Here's how the part is built. I have some questions about the finished solid (model axes, mm). Round coordinates to 2 decimals unless told otherwise and drop trailing zeros. Order: outer loops, then holes, each group sorted by start corner. A loop starts at its lowest first (then second) coordinate and runs counter-clockwise, first axis right, second up. Notation, with made-up numbers: (55.5, 85.25) -> (67.5, 85.25) arc R26 ccw to (67.5, 114.25) -> close; hole circle Ø3 at (14.5, -13). An arc over 180 degrees is marked (long way). Answer in a Markdown table with one row per item.
```python
from build123d import *

# Parameters (mm, degrees)
SKETCH1_W           = 16
SKETCH1_H           = 20
BOSS_EXTRUDE1_DEPTH = 4.2
SKETCH2_R           = 2.25
CUT_EXTRUDE1_DEPTH  = 26.954575704
FILLET1_R           = 8


with BuildPart() as part:
    # Sketch1 → Boss-Extrude1 (new body)
    with BuildSketch(Plane.XY):
        with Locations((8, 10)):
            Rectangle(SKETCH1_W, SKETCH1_H)
    extrude(amount=BOSS_EXTRUDE1_DEPTH)

    # Sketch2 → Cut-Extrude1 (cut, through all)
    with BuildSketch(Plane.XY.offset(4.2)):
        with Locations((8, 10.8)):
            Circle(SKETCH2_R)
    extrude(amount=-CUT_EXTRUDE1_DEPTH, mode=Mode.SUBTRACT)

    # Fillet1
    fillet1_edges = [part.edges().sort_by_distance(p)[0] for p in [
        (16, 20, 2.1),
        (0, 20, 2.1),
    ]]
    fillet(fillet1_edges, radius=FILLET1_R - 0.0001)  # a hair under: the kernel refuses the full size


solid = part.part
```
1. Suppose I cut it at C-C on x = 6.5. Write out the boundary of the cut face in (y, z).
Numbers:
| item | result |
|---|---|
| outline | (0, 0) -> (9.12, 0) -> (9.12, 4.2) -> (0, 4.2) -> close; (12.48, 0) -> (19.86, 0) -> (19.86, 4.2) -> (12.48, 4.2) -> close |
2. We'd pull the mould along X, two halves only. Please class faces 1 (the face through (8, 8, 4.2)), 2 (the face through (6.34, 12.32, 2.13)), 3 (the face through (2.281, 17.594, 2.129)): released by +X, released by -X, zero draft, split by the parting line, or undercut.
Numbers:
| item | result |
|---|---|
| face 1 | zero draft |
| face 2 | undercut |
| face 3 | released by -X |
3. Suppose I cut it at A-A on y = 10.8. Write out the boundary of the cut face in (x, z).
Numbers:
| item | result |
|---|---|
| outline | (0, 0) -> (5.75, 0) -> (5.75, 4.2) -> (0, 4.2) -> close; (10.25, 0) -> (16, 0) -> (16, 4.2) -> (10.25, 4.2) -> close |
4. Suppose I cut it at D-D on y = 17.5. Write out the boundary of the cut face in (x, z).
Numbers:
| item | result |
|---|---|
| outline | (2.19, 0) -> (13.81, 0) -> (13.81, 4.2) -> (2.19, 4.2) -> close |
5. Please list where these lines run through material, in increasing order: line 1 along Y through (x, z) = (8, 3.1); line 2 along Y through (x, z) = (10, 0.3); line 3 along Y through (x, z) = (12.25, 1.75).
Numbers:
| item | result |
|---|---|
| line 1 | y = 0 to 8.55, 13.05 to 20 |
| line 2 | y = 0 to 9.77, 11.83 to 19.75 |
| line 3 | y = 0 to 18.78 |
